Here's how the part is built. I have some questions about the finished solid (model axes, mm). A direction names the side the tool comes from. Round coordinates to 2 decimals unless told otherwise and drop trailing zeros. Write each loop counter-clockwise with the first axis right and the second up, starting at its lowest first coordinate (ties: lowest second). Pieces come first, ordered by that corner, then holes. Notation, with made-up numbers: (-3.5, -39.5) - (26.5, -39.5) arc R19 ccw to (26.5, -15.5) - close; hole circle Ø9 at (40.25, 0). An arc over 180 degrees is marked (long way). One line per question, with ' | ' between items. Start each with the question number.
(1) Will these pins go through, and if not, where does the flat tip stop? pin 1 (5 mm diameter, centred on x = 5.5, y = 27, fed in from -Z); pin 2 (8 mm diameter, centred on x = -1, y = 51.5, fed in from +Z); pin 3 (12 mm diameter, centred on x = -20, y = 17.5, fed in from +Z); pin 4 (1.5 mm diameter, centred on x = -2.5, z = 3.5, fed in from +Y).
(2) Imagine slicing it at B-B (z = -3). Write out the boundary of the cut face in (x, y).
(3) Thinking about a two-plate mould opening in X: for faces 3 (the cylindrical face through (5.506, 37.567, 24.796)), 4 (the flat face through (0.651, 38.633, 6.317)), 5 (the flat face through (-5, 0, -5)), which applies, pulls with the +X half, pulls with the -X half, needs draft (parallel to the pull), parting line crosses it, or undercut?
(4) Imagine slicing it at A-A (x = 1). Write out the boundary of the cut face in (y, z).
(5) If I drill on L1, parallel to X at y = 46.5, z = 4; L2, parallel to X at y = 58.5, z = 5; L3, parallel to Z at x = 5.5, y = 40, over which ranges is the centre line in solid material (lowest first)?
(6) Imagine slicing it at D-D (z = 18). Write out the boundary of the cut face in (x, y).
(7) For faces 1 (the flat face through (5.8, 38.63, 2.59)), 2 (the flat face through (-5, 76.2, -5)), which set-ups out of +Z, -Z, +X, -X, +Y, -Y let a thin tool reach every point of the face, with its end or its side?
(8) Imagine slicing it at C-C (y = 21). Write out the boundary of the cut face in (x, z).
Autodesk Inventor part; units mm, degrees
ref_plane "YZ Plane" through (0, 0, 0) normal (1, 0, 0) x (0, 1, 0)
ref_plane "XZ Plane" through (0, 0, 0) normal (0, 1, 0) x (-1, 0, 0)
ref_plane "XY Plane" through (0, 0, 0) normal (0, 0, 1) x (1, 0, 0)
sketch "Sketch1" plane through (0, 0, 0) normal (0, 1, 0) x (-1, 0, 0)
  circle A0 centre (0, 0) radius 25.4
  dimension "d0" = 50.8
extrude "Extrusion1" add sketch "Sketch1" along normal blind 76.2
sketch "Sketch2" plane through (0, 76.2, 0) normal (0, 1, 0) x (1, 0, 0)
  line L0 (4.2496, -5.9753) -> (-3.0499, -6.6679)
  line L1 (-3.0499, -6.6679) -> (-7.2996, -0.6926)
  line L2 (-7.2996, -0.6926) -> (-4.2496, 5.9753)
  line L3 (-4.2496, 5.9753) -> (3.0499, 6.6679)
  line L4 (3.0499, 6.6679) -> (7.2996, 0.6926)
  line L5 (7.2996, 0.6926) -> (4.2496, -5.9753)
  point P0 (0, 0)
  point P1 (0, 0)
  dimension "d3" = 12.7
extrude "Extrusion2" cut sketch "Sketch2" against normal through all
Check sheet entries:
1) pin 1: z = -25.22 | pin 2: z = 25.4 | pin 3: z = 21.19 | pin 4: through
2) outline: (-25.22, 0) - (-5.61, 0) - (-5.61, 76.2) - (-25.22, 76.2) - close; (5.66, 0) - (25.22, 0) - (25.22, 76.2) - (5.66, 76.2) - close
3) face 3: parting line crosses it | face 4: undercut | face 5: needs draft
4) outline: (0, -25.38) - (76.2, -25.38) - (76.2, -6.47) - (0, -6.47) - close; (0, 6.28) - (76.2, 6.28) - (76.2, 25.38) - (0, 25.38) - close
5) L1: -25.08 to -4.95, 5.15 to 25.08 | L2: -24.9 to -4.24, 4.7 to 24.9 | L3: -24.8 to -3.22, 3.24 to 24.8
6) outline: (-17.92, 0) - (17.92, 0) - (17.92, 76.2) - (-17.92, 76.2) - close
7) face 1: +Y, -Y | face 2: +Z, -Z, +X, -X, +Y
8) outline: circle Ø50.8 at (0, 0); hole (-7.3, 0.69) - (-4.25, -5.98) - (3.05, -6.67) - (7.3, -0.69) - (4.25, 5.98) - (-3.05, 6.67) - close
